Autodesk Fusion 360 part; units mm, degrees
sketch "Esquisse1" plane through (0, 0, 0) normal (0, 0, 1) x (1, 0, 0)
  circle A0 centre (0, 0) radius 6
  dimension "d1" = 12
extrude "Extrusion1" add sketch "Esquisse1" along normal blind 117
sketch "Esquisse2" plane through (0, 0, 117) normal (0, 0, 1) x (-1, 0, 0)
  circle A0 centre (0, 0) radius 6
  circle A1 centre (0, 0) radius 2.5
  dimension "d5" = 5
extrude "Extrusion2" cut sketch "Esquisse2" against normal blind 12 contours A1
sketch "Esquisse3" plane through (0, 0, 0) normal (0, 0, -1) x (1, 0, 0)
  circle A0 centre (0, 0) radius 6
  circle A1 centre (0, 0) radius 2.5
  dimension "d8" = 5
extrude "Extrusion3" cut sketch "Esquisse3" against normal blind 12 contours A1
sketch "Esquisse4" plane through (0, 0, 117) normal (0, 0, 1) x (-1, 0, 0)
  circle A0 centre (0, 0) radius 2.5
  circle A1 centre (0, 0) radius 6
  line L0 (5, 8) -> (-5, 8)
  line L1 (-5, 8) -> (-5, -7.4606)
  line L2 (-5, -7.4606) -> (5, -7.4606)
  line L3 (5, -7.4606) -> (5, 8)
  dimension "d11" = 5
  dimension "d12" = 10
extrude "Extrusion4" cut sketch "Esquisse4" against normal blind 10 from surface at -20 contours A1 L3 | A1 L1
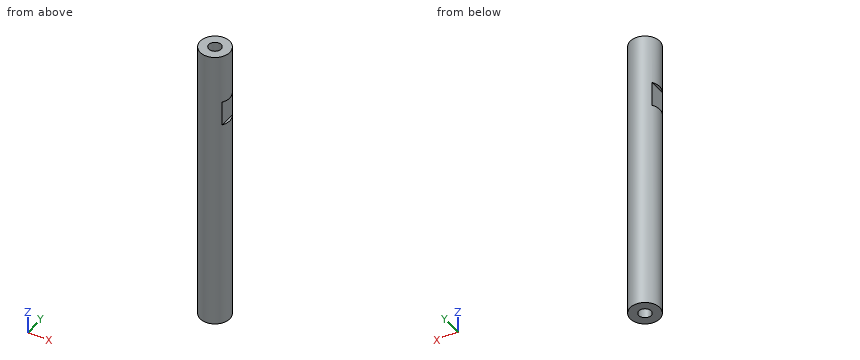
Check sheet for the modelled part. Datum: model origin and axes. Units: mm. Give positions to 0.01 mm unless a question says otherwise; leave off trailing zeros. Write each loop counter-clockwise with the first axis right and the second up, starting at its lowest first coordinate (ties: lowest second). Pieces come first, ordered by that corner, then holes. Notation, with made-up numbers: (69, -25) -> (109, -25) arc R17 ccw to (109, -16) -> close; hole circle Ø10 at (-16, 41). An arc over 180 degrees is marked (long way). Write item = value, one per line.
Item 1: Sectioned sample at B-B on x = 0. Record the boundary of the cut face in (y, z).
Output:
outline = (-6, 0) -> (-2.5, 0) -> (-2.5, 12) -> (2.5, 12) -> (2.5, 0) -> (6, 0) -> (6, 117) -> (2.5, 117) -> (2.5, 105) -> (-2.5, 105) -> (-2.5, 117) -> (-6, 117) -> close
Item 2: Sectioned sample at C-C on z = 94. Record the boundary of the cut face in (x, y).
Output:
outline = (-5, -3.32) arc R6 ccw to (5, -3.32) -> (5, 3.32) arc R6 ccw to (-5, 3.32) -> close
Item 3: Sectioned sample at D-D on y = -5. Record the boundary of the cut face in (x, z).
Output:
outline = (-3.32, 0) -> (3.32, 0) -> (3.32, 117) -> (-3.32, 117) -> close
Item 4: Gauge pin test, flat ends, axial feed: pin 1 (4 mm diameter, centred on x = -0.5, y = 0.5, fed in from -Z); pin 2 (3.5 mm diameter, centred on y = -1.5, z = 90.5, fed in from +X); pin 3 (1 mm diameter, centred on x = 1, z = 59.5, fed in from +Y); pin 4 (2 mm diameter, centred on y = 1.5, z = 92.5, fed in from -X). Record the tip position at first contact, or that the pin passes through.
Output:
pin_1 = 0
pin_2 = 5
pin_3 = 5.98
pin_4 = -5
Item 5: Scan lines: probe 1 along X at (y, z) = (0, 108.5); probe 2 along X at (y, z) = (-0.25, 101.5). Record each from-to range of solid material in increasing order. Write a range as from..to.
Output:
probe_1 = -6..-2.5, 2.5..6
probe_2 = -5.99..5.99
Item 6: Sectioned sample at A-A on y = 0. Record the boundary of the cut face in (x, z).
Output:
outline = (-6, 0) -> (-2.5, 0) -> (-2.5, 12) -> (2.5, 12) -> (2.5, 0) -> (6, 0) -> (6, 87) -> (5, 87) -> (5, 97) -> (6, 97) -> (6, 117) -> (2.5, 117) -> (2.5, 105) -> (-2.5, 105) -> (-2.5, 117) -> (-6, 117) -> (-6, 97) -> (-5, 97) -> (-5, 87) -> (-6, 87) -> close
